Design review of the part shown in the three views and the two pictorial views. Dimensions are in mm from the part's minimum x, y and z. Round coordinates to 2 decimals unless told otherwise and drop trailing zeros. Order: outer loops, then holes, each group sorted by start corner. A loop starts at its lowest first (then second) coordinate and runs counter-clockwise, first axis right, second up. Notation, with made-up numbers: M 19.25,18.5 L 74.25,18.5 A16 cw 74.25,23.5 Z; hole C 3,42 d3. An arc over 180 degrees is marked long. Write each question's results on one line, items separated by ' | '. Start each with the question number.
Item 1: Take a section at D-D, the plane z = 3.5. Write out the cut boundary in (x, y), plus the area to 3 significant figures.
Item 2: Take a section at A-A, the plane z = 5.75. Write out the cut boundary in (x, y).
Item 3: Take a section at B-B, the plane y = 0.4. Write out the cut boundary in (x, z) (3 decimals), plus the area to 3 significant figures.
Item 4: Wall thickness on line 1 (X direction, y = 0.35, z = 6); line 2 (X direction, y = 0.45, z = 5.5); line 3 (Z direction, x = 5.5, y = 0.1): over which ranges is each line inside the solid? List them lowest first. Write a range as [from, to].
Item 5: Take a section at C-C, the plane x = 4.5. Write out the cut boundary in (y, z).
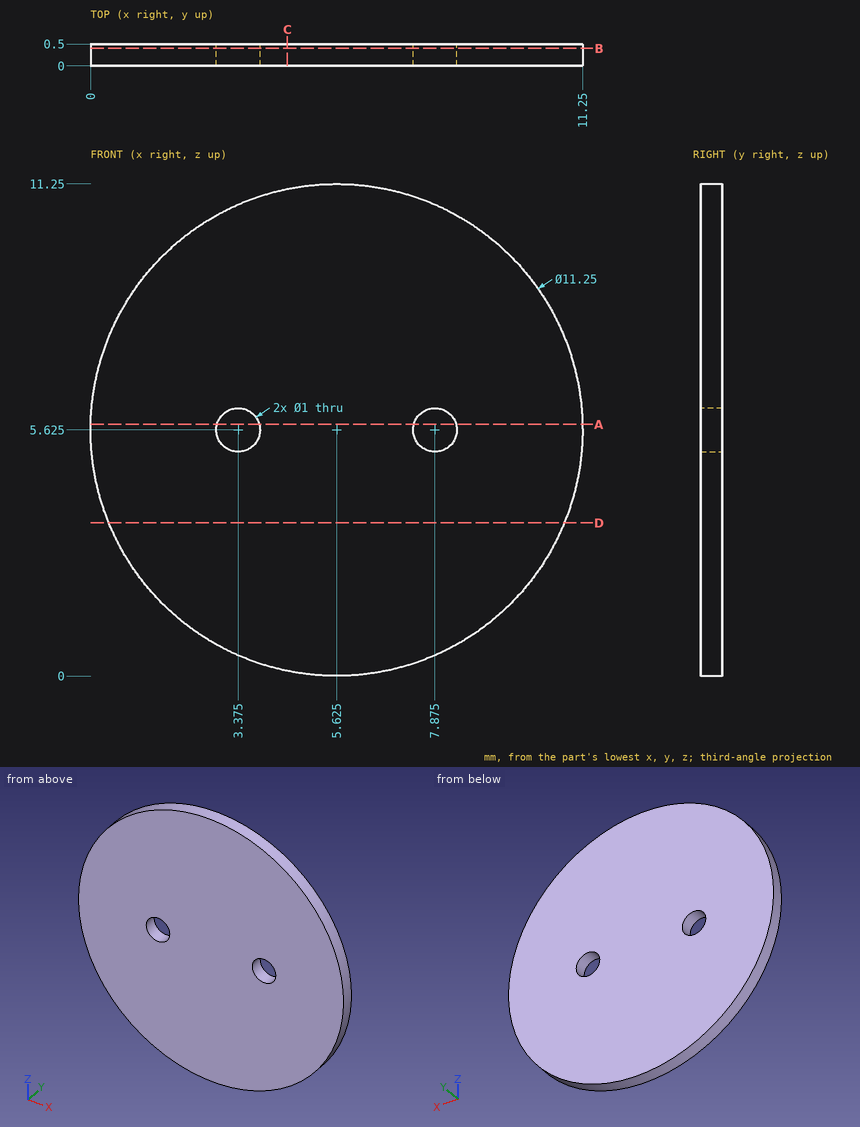
Results list:
1) outline: M 0.42,0 L 10.83,0 L 10.83,0.5 L 0.42,0.5 Z | area: 5.21 mm²
2) outline: M 0,0 L 2.89,0 L 2.89,0.5 L 0,0.5 Z; M 3.86,0 L 7.39,0 L 7.39,0.5 L 3.86,0.5 Z; M 8.36,0 L 11.25,0 L 11.25,0.5 L 8.36,0.5 Z
3) outline: C 5.625,5.625 d11.25; hole C 3.375,5.625 d1; hole C 7.875,5.625 d1 | area: 97.8 mm²
4) line 1: [0.01, 3.04], [3.71, 7.54], [8.21, 11.24] | line 2: [0, 2.89], [3.86, 7.39], [8.36, 11.25] | line 3: [0, 11.25]
5) outline: M 0,0.11 L 0.5,0.11 L 0.5,11.14 L 0,11.14 Z
